Could you check a few things on this model? Use its own coordinates, in mm. Give positions to 0.01 mm unless a question says otherwise; leave off trailing zeros. Write each loop counter-clockwise with the first axis right and the second up, starting at its lowest first coordinate (ties: lowest second). Pieces come first, ordered by that corner, then holes. Notation, with made-up numbers: (14.5, -39) - (38.5, -39) arc R32 ccw to (38.5, 0) - close; hole circle Ø7 at (88, 35). An arc over 180 degrees is marked (long way). Answer in a Markdown table with one row per item.
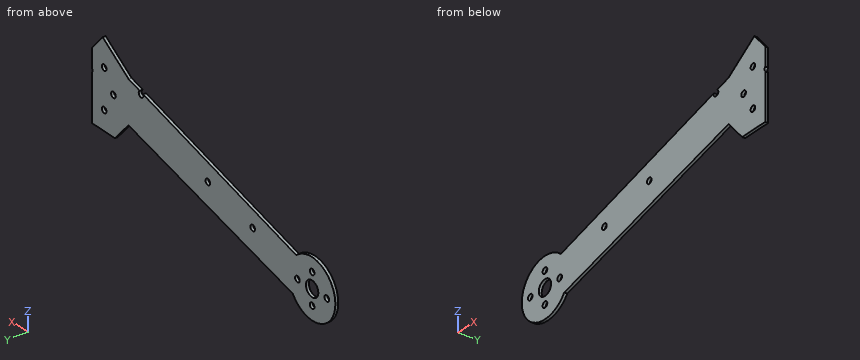
from build123d import *

# Parameters (mm, degrees)
SKETCH1_R           = 1.5
SKETCH1_R_2         = 4
BOSS_EXTRUDE1_DEPTH = 1.5


with BuildPart() as part:
    # Sketch1 → Boss-Extrude1 (new body)
    with BuildSketch(Plane(origin=(0, 0, 0), x_dir=(1, 0, 0), z_dir=(0, 1, 0))):
        with BuildLine():
            Line((-7.070663707, -8.426488874), (0, 0))
            Line((0, 0), (0, 9.381966011))
            ThreePointArc((0, 9.381966011), (-0.5, 10.5), (0, 11.618033989))
            Line((0, 11.618033989), (0, 35.5))
            Line((0, 35.5), (-15, 35.5))
            Line((-15, 35.5), (-23.677632731, 25.158400018))
            Line((-23.677632731, 25.158400018), (-129.929473623, 53.628494979))
            ThreePointArc((-129.929473623, 53.628494979), (-157.327989791, 47.078833109), (-132.17932297, 34.38547595))
            Line((-132.17932297, 34.38547595), (-33.223789423, 6.015437425))
            ThreePointArc((-33.223789423, 6.015437425), (-31.446611343, 8.081911862), (-31.03429168, 5.387719772))
            Line((-31.03429168, 5.387719772), (-23.863280614, 3.331828071))
            Line((-23.863280614, 3.331828071), (-7.070663707, -8.426488874))
        make_face()
        with Locations(Location((-8, 5.5, 0), (0, 0, 270))):
            Circle(SKETCH1_R, mode=Mode.SUBTRACT)
        with Locations(Location((-14, 15.5, 0), (0, 0, 270))):
            Circle(SKETCH1_R, mode=Mode.SUBTRACT)
        with Locations(Location((-8, 25.5, 0), (0, 0, 270))):
            Circle(SKETCH1_R, mode=Mode.SUBTRACT)
        with Locations(Location((-142.429473623, 37.336933003, 0), (0, 0, 270))):
            Circle(SKETCH1_R, mode=Mode.SUBTRACT)
        with Locations(Location((-104.014603511, 35.04369958, 0), (0, 0, 270))):
            Circle(SKETCH1_R, mode=Mode.SUBTRACT)
        with Locations(Location((-151.929473623, 45.336933003, 0), (0, 0, 270))):
            Circle(SKETCH1_R, mode=Mode.SUBTRACT)
        with Locations(Location((-142.429473623, 45.336933003, 0), (0, 0, 270))):
            Circle(SKETCH1_R_2, mode=Mode.SUBTRACT)
        with Locations(Location((-132.929473623, 45.336933003, 0), (0, 0, 270))):
            Circle(SKETCH1_R, mode=Mode.SUBTRACT)
        with Locations(Location((-142.429473623, 53.336933003, 0), (0, 0, 270))):
            Circle(SKETCH1_R, mode=Mode.SUBTRACT)
        with Locations(Location((-75.036828722, 27.279128226, 0), (0, 0, 270))):
            Circle(SKETCH1_R, mode=Mode.SUBTRACT)
    extrude(amount=BOSS_EXTRUDE1_DEPTH)


solid = part.part
1) If I drill on line 1 (Z direction, x = -105, y = 0.3); line 2 (Z direction, x = -106.5, y = 0.55); line 3 (X direction, y = 1.2, z = 0), over which ranges is the centre line in solid material (lowest first)?
Check values:
| item | result |
|---|---|
| line 1 | z = -46.95 to -36.17, -33.91 to -26.59 |
| line 2 | z = -47.35 to -27.02 |
| line 3 | x = -19.1 to 0 |
2) Will these pins go through, and if not, where does the flat tip stop? P1, Ø6.5, axis at x = -142.43, z = -45.34, coming from the +Y side; P2, Ø0.8, axis at x = -10.5, y = 0.5, coming from the -Z side.
Check values:
| item | result |
|---|---|
| P1 | passes through |
| P2 | stops at z = -35.5 |
3) Imagine slicing it at A-A (z = -15.5). List the corners of the cut face in (x, y) for me.
Check values:
| item | result |
|---|---|
| outline | (-66.31, 0) - (-15.5, 0) - (-15.5, 1.5) - (-66.31, 1.5) - close; (-12.5, 0) - (0, 0) - (0, 1.5) - (-12.5, 1.5) - close |
4) Imagine slicing it at D-D (x = -43). List the corners of the cut face in (y, z) for me, then the cut area to 3 significant figures.
Check values:
| item | result |
|---|---|
| outline | (0, -30.34) - (1.5, -30.34) - (1.5, -8.82) - (0, -8.82) - close |
| area | 32.3 mm2 |
5) Imagine slicing it at B-B (y = 0.3). State how many separate pieces and enclosed holes the cut face has, then the cut area to 3 significant figures.
Check values:
| item | result |
|---|---|
| separate pieces | 1 |
| enclosed holes | 10 |
| area | 3,650 mm2 |
6) Imagine slicing it at C-C (x = -61.5). List the corners of the cut face in (y, z) for me.
Check values:
| item | result |
|---|---|
| outline | (0, -35.29) - (1.5, -35.29) - (1.5, -14.12) - (0, -14.12) - close |
